Here's how the part is built. I have some questions about the finished solid (model axes, mm). Round coordinates to 2 decimals unless told otherwise and drop trailing zeros. Write each loop counter-clockwise with the first axis right and the second up, starting at its lowest first coordinate (ties: lowest second). Pieces come first, ordered by that corner, then holes. Notation, with made-up numbers: M 6,-10.5 L 18,-10.5 A13 ccw 18,1.5 Z; hole C 40.25,-26.75 d6. An arc over 180 degrees is marked long. Use a Markdown table: item, result. Add a question column.
```python
from build123d import *

# Parameters (mm, degrees)
BOX003_W        = 25
BOX003_H        = 2900
BOX003_DEPTH    = 70
CHAMFER_SIZE    = 20
CHAMFER001_SIZE = 20


with BuildPart() as part:
    # Box003 → Box003 (new body)
    with BuildSketch(Plane(origin=(200, 0, 0), x_dir=(1, 0, 0), z_dir=(0, 0, 1))):
        with Locations((12.5, 1450)):
            Rectangle(BOX003_W, BOX003_H)
    extrude(amount=BOX003_DEPTH)

    # Chamfer
    chamfer_edges = [part.edges().sort_by_distance(p)[0] for p in [
        (225, 1450, 70),
    ]]
    chamfer(chamfer_edges, length=CHAMFER_SIZE)

    # Chamfer001
    chamfer001_edges = [part.edges().sort_by_distance(p)[0] for p in [
        (200, 1450, 0),
    ]]
    chamfer(chamfer001_edges, length=CHAMFER001_SIZE)


with BuildPart() as part_1:
    # Chamfer001 placement: moved
    add(part.part.moved(Location((-140, 100, 10))))


solid = part_1.part
```
Item 1: Imagine slicing it at B-B on x = 74.25. List the corners of the cut face in (y, z) for me, plus the area to 4 significant figures.
Item 2: I need wall thicknesses on probe 1 along Z at (x, y) = (79.5, 1924); probe 2 along Z at (x, y) = (83.5, 1962.5); probe 3 along X at (y, z) = (2634, 72). Which ranges of each line are inside material? Lowest first, please. Write a range as from..to.
Item 3: Imagine slicing it at A-A on y = 357. List the corners of the cut face in (x, z) for me.
The answers:
| question | item | result |
|---|---|---|
| 1 | outline | M 100,15.75 L 3000,15.75 L 3000,70.75 L 100,70.75 Z |
| 1 | area | 159,500 mm² |
| 2 | probe 1 | 10.5..65.5 |
| 2 | probe 2 | 10..61.5 |
| 2 | probe 3 | 60..73 |
| 3 | outline | M 60,30 L 80,10 L 85,10 L 85,60 L 65,80 L 60,80 Z |
